Here's how the part is built. I have some questions about the finished solid (model axes, mm). Face numbers are marked on the shaded views. A direction names the side the tool comes from. Coordinates: 2 decimals unless noted, no trailing zeros. Order: outer loops, then holes, each group sorted by start corner. A loop starts at its lowest first (then second) coordinate and runs counter-clockwise, first axis right, second up. Notation, with made-up numbers: M -0.5,-31 L 44.5,-31 A11 ccw 44.5,-23 Z; hole C -29,-36 d2. An arc over 180 degrees is marked long. Answer as CSV lines item,"result". Start each with the question number.
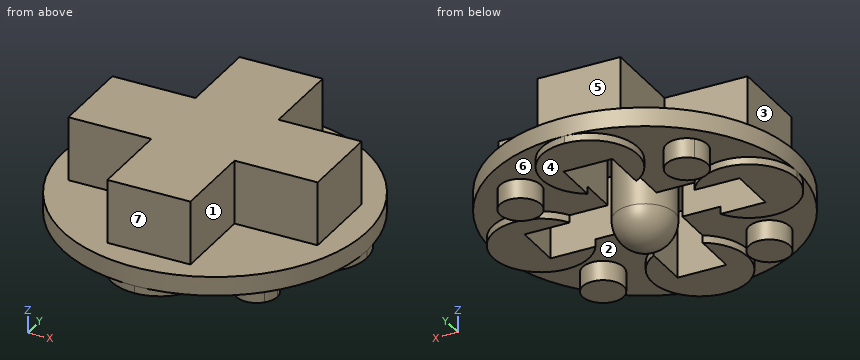
```python
from build123d import *

# Parameters (mm, degrees)
F0_R      = 12.8
F1_DEPTH  = 1.6
F2_W      = 7
F2_H      = 7
F3_DEPTH  = 5.38
F4_W      = 4.11
F4_H      = 7
F4_W_2    = 7
F4_H_2    = 4.11
F5_DEPTH  = 5
F6_R      = 2.5
F7_DEPTH  = 8.3
F9_DEPTH  = 0.63
F11_DEPTH = 1.65
F12_R     = 2.5


with BuildPart() as f1:
    # F0 (on Top) → F1 (new body)
    with BuildSketch(Plane.XY):
        Circle(F0_R)
    extrude(amount=F1_DEPTH)

    # F2 (on face) → F3 (join)
    with BuildSketch(Plane.XY.offset(1.6)):
        with Locations((0, 7)):
            Rectangle(F2_W, F2_H)
        with Locations((7, 0)):
            Rectangle(F2_W, F2_H)
        Rectangle(F2_W, F2_H)
        with Locations((-7, 0)):
            Rectangle(F2_W, F2_H)
        with Locations((0, -7)):
            Rectangle(F2_W, F2_H)
    extrude(amount=F3_DEPTH)

    # F4 (on face) → F5 (cut)
    with BuildSketch(Plane(origin=(0, 0, 0), x_dir=(1, 0, 0), z_dir=(0, 0, -1))):
        with Locations((0, -5.555)):
            Rectangle(F4_W, F4_H)
        with Locations((-5.555, 0)):
            Rectangle(F4_W_2, F4_H_2)
        Rectangle(F4_W, F4_H_2)
        with Locations((5.555, 0)):
            Rectangle(F4_W_2, F4_H_2)
        with Locations((0, 5.555)):
            Rectangle(F4_W, F4_H)
    extrude(amount=-F5_DEPTH, mode=Mode.SUBTRACT)

    # F6 (on face) → F7 (join)
    with BuildSketch(Plane(origin=(0, 0, 5), x_dir=(1, 0, 0), z_dir=(0, 0, -1))):
        Circle(F6_R)
    extrude(amount=F7_DEPTH)

    # F8 (on face) → F9 (join)
    with BuildSketch(Plane(origin=(0, 0, 0), x_dir=(1, 0, 0), z_dir=(0, 0, -1))):
        with BuildLine():
            ThreePointArc((-5.2600895427, 2.055), (-9.8149794946, 3.9074696001), (-12.8, 0))
            ThreePointArc((-12.8, 0), (-9.8149794946, -3.9074696001), (-5.2600895427, -2.055))
            Line((-5.2600895427, -2.055), (-9.055, -2.055))
            Line((-9.055, -2.055), (-9.055, 2.055))
            Line((-9.055, 2.055), (-5.2600895427, 2.055))
        make_face()
        with BuildLine():
            ThreePointArc((2.055, 5.2600895427), (3.516052474, 6.7400559709), (4.05, 8.75))
            ThreePointArc((4.05, 8.75), (2.8637824638, 11.6137824638), (0, 12.8))
            ThreePointArc((0, 12.8), (-3.9074696001, 9.8149794946), (-2.055, 5.2600895427))
            Line((-2.055, 5.2600895427), (-2.055, 9.055))
            Line((-2.055, 9.055), (2.055, 9.055))
            Line((2.055, 9.055), (2.055, 5.2600895427))
        make_face()
        with BuildLine():
            ThreePointArc((5.2600895427, -2.055), (9.8149794946, -3.9074696001), (12.8, 0))
            ThreePointArc((12.8, 0), (9.8149794946, 3.9074696001), (5.2600895427, 2.055))
            Line((5.2600895427, 2.055), (9.055, 2.055))
            Line((9.055, 2.055), (9.055, -2.055))
            Line((9.055, -2.055), (5.2600895427, -2.055))
        make_face()
        with BuildLine():
            ThreePointArc((-2.055, -5.2600895427), (-3.9074696001, -9.8149794946), (0, -12.8))
            ThreePointArc((0, -12.8), (2.8637824638, -11.6137824638), (4.05, -8.75))
            ThreePointArc((4.05, -8.75), (3.516052474, -6.7400559709), (2.055, -5.2600895427))
            Line((2.055, -5.2600895427), (2.055, -9.055))
            Line((2.055, -9.055), (-2.055, -9.055))
            Line((-2.055, -9.055), (-2.055, -5.2600895427))
        make_face()
    extrude(amount=F9_DEPTH)

    # F10 (on face) → F11 (join)
    with BuildSketch(Plane(origin=(0, 0, 0), x_dir=(1, 0, 0), z_dir=(0, 0, -1))):
        with BuildLine():
            ThreePointArc((-7.9112882596, 8.3463475889), (-7.4059830041, 5.5096760997), (-4.9995950218, 7.0943954494))
            ThreePointArc((-4.9995950218, 7.0943954494), (-6.0432070395, 8.6791147992), (-7.9112882596, 8.3463475889))
        make_face()
        with BuildLine():
            ThreePointArc((-5.3693954494, -6.7245950218), (-7.7331471854, -5.1222151605), (-8.3463475884, -7.91128826))
            ThreePointArc((-8.3463475884, -7.91128826), (-6.4556437135, -8.3269748831), (-5.3693954494, -6.7245950218))
        make_face()
        with BuildLine():
            ThreePointArc((8.4495950218, -7.0943954494), (5.1398756712, -6.4130074691), (7.9112882626, -8.346347586))
            ThreePointArc((7.9112882626, -8.346347586), (8.3093143724, -7.7757834298), (8.4495950218, -7.0943954494))
        make_face()
        with BuildLine():
            ThreePointArc((8.8193954494, 6.7245950218), (8.6967753098, 7.36334676), (8.3463475851, 7.9112882636))
            ThreePointArc((8.3463475851, 7.9112882636), (5.492015589, 6.0858432836), (8.8193954494, 6.7245950218))
        make_face()
    extrude(amount=F11_DEPTH)

    # F12
    f12_edges = [f1.edges().sort_by_distance(p)[0] for p in [
        (-2.5, 0, -3.3),
    ]]
    fillet(f12_edges, radius=F12_R)


solid = f1.part
```
1) If we mould it in two halves opening along X, with no side actions, what happens to the marked faces 1, 2, 3 and 4? For each: released by +X, released by -X, zero draft, split by the parting line, or undercut.
2) Suppose I cut it at B-B on z = 6. Please give me the cut outline in (x, y).
3) Will these pins go through, and if not, where does the flat tip stop? pin 1 Ø2.5 at (y, z) = (1.5, 4) entering from +X; pin 2 Ø1.5 at (x, z) = (8.5, 4.5) entering from +Y; pin 3 Ø4.5 at (y, z) = (6, 2.5) entering from -X.
4) Suppose I cut it at C-C on x = -6. Please give me the cut outline in (y, z) (3 decimals).
5) I need wall thicknesses on line 1 (Y direction, x = -9, z = 4.5) (3 decimals); line 2 (Z direction, x = -2.5, y = -5.75); line 3 (Z direction, x = -0.75, y = -8.5). Which ranges of each line are inside material? Lowest first, please. Write a range as [from, to].
6) Suppose I cut it at A-A on z = 0.75. Please give me the cut outline in (x, y) (3 decimals), plus the area to 3 significant figures.
7) Which directions (+Z, -Z, +X, -X, +Y, -Y) give clear straight access to the entire face, cutting with the end or side of a thin tool? Please do the marked faces 5, 6 and 7.
Output:
1,face 1,"released by +X"
1,face 2,"undercut"
1,face 3,"released by -X"
1,face 4,"undercut"
2,outline,"M -10.5,-3.5 L -3.5,-3.5 L -3.5,-10.5 L 3.5,-10.5 L 3.5,-3.5 L 10.5,-3.5 L 10.5,3.5 L 3.5,3.5 L 3.5,10.5 L -3.5,10.5 L -3.5,3.5 L -10.5,3.5 Z"
3,pin 1,"x = 10.5"
3,pin 2,"y = 3.5"
3,pin 3,"x = -12.18"
4,outline,"M -11.307,0 L -8.66,0 L -8.66,-1.65 L -5.529,-1.65 L -5.529,0 L -2.973,0 L -2.973,-0.63 L -2.055,-0.63 L -2.055,5 L 2.055,5 L 2.055,-0.63 L 2.973,-0.63 L 2.973,0 L 5.391,0 L 5.391,-1.65 L 8.058,-1.65 L 8.058,0 L 11.307,0 L 11.307,1.6 L 3.5,1.6 L 3.5,6.98 L -3.5,6.98 L -3.5,1.6 L -11.307,1.6 Z"
5,line 1,"[-3.5, -2.055], [2.055, 3.5]"
5,line 2,"[-0.63, 6.98]"
5,line 3,"[5, 6.98]"
6,outline,"C 0,0 d25.6; C 0,0 d5; hole M -9.055,-2.055 L -2.055,-2.055 L -2.055,-9.055 L 2.055,-9.055 L 2.055,-2.055 L 9.055,-2.055 L 9.055,2.055 L 2.055,2.055 L 2.055,9.055 L -2.055,9.055 L -2.055,2.055 L -9.055,2.055 Z"
6,area,"402 mm²"
7,face 5,"+Z, +X, -X, +Y"
7,face 6,"-Z"
7,face 7,"+Z, +X, -X, -Y"
